Geometry: see drawing. Coordinates: mm, zero at the bounding-box minimum. A direction names the side the tool comes from. Round coordinates to 2 decimals unless told otherwise and drop trailing zeros. Loops run counter-clockwise (first coordinate to the right, second up) from the corner with the lowest first, then second, coordinate; pieces in that order, holes last.
(1) Cut plane A-A, the plane x = 4.75. Output: boundary loops of the cut face in (y, z).
(2) Draft query along X for the marked faces 3, 4, 5 and 6. Return one class per face: released by +X, released by -X, zero draft, split by the parting line, or undercut.
(3) First-contact query: pin 1 Ø1.5 at (x, y) = (9, 34.5) entering from -Z; pin 2 Ø5 at (x, y) = (8, 24.5) entering from +Z; pin 3 Ø1.5 at (x, z) = (8, 1.5) entering from +Y. Flat tips, straight axial feed; report the tip coordinate or a pass-through.
(4) Cut plane B-B, the plane z = 3.75. Output: boundary loops of the cut face in (x, y), and give its area (3 significant figures).
(5) Access query for the marked faces 1 and 2. Directions: +Z, -Z, +X, -X, +Y, -Y. A direction counts if a zero-diameter tool reaches every point of the face in a straight line with its end or side. Return the directions, or none.
(6) Line query: line 1 (Z direction, x = 3.25, y = 8); line 2 (X direction, y = 16.5, z = 4); line 3 (Z direction, x = 14.25, y = 33.5). Output: solid intervals per line, ascending.
(7) Cut plane D-D, the plane x = 14.75. Output: boundary loops of the cut face in (y, z).
(8) Cut plane C-C, the plane y = 35. Output: boundary loops of the cut face in (x, z), and give its area (3 significant figures).
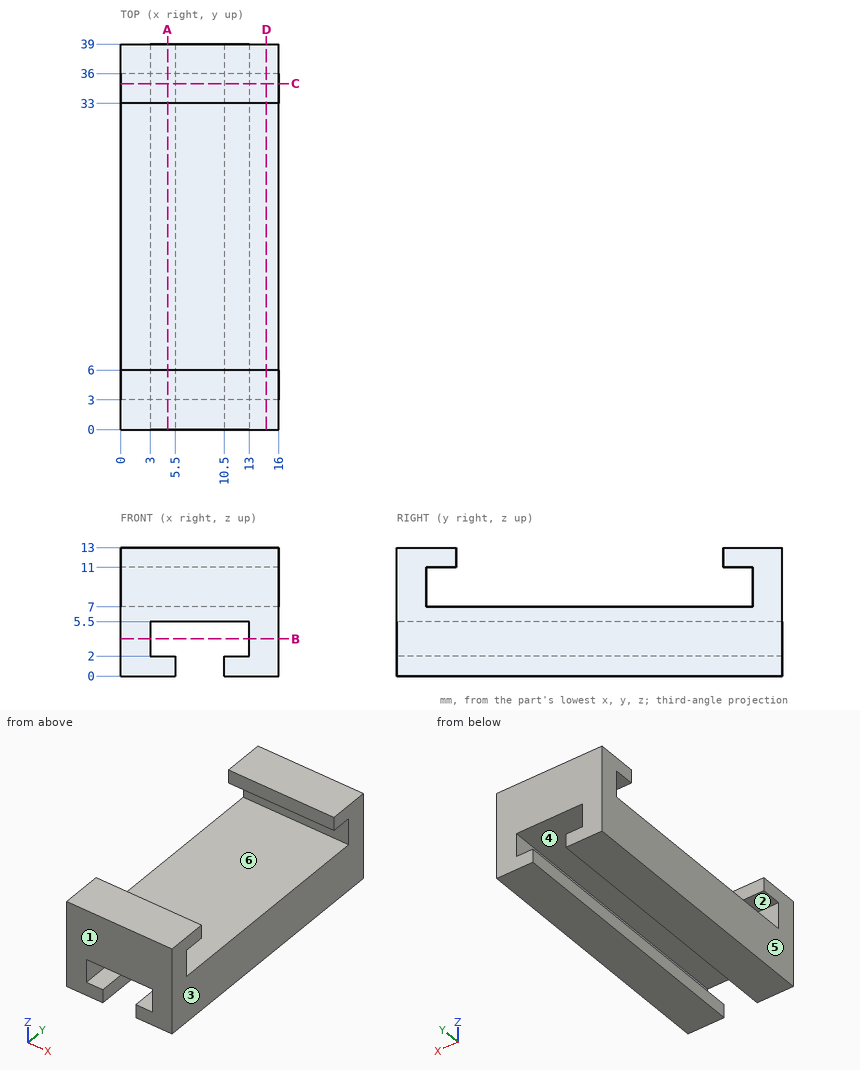
Reported:
1. outline: (0, 0) - (39, 0) - (39, 2) - (0, 2) - close; (0, 5.5) - (39, 5.5) - (39, 13) - (33, 13) - (33, 11) - (36, 11) - (36, 7) - (3, 7) - (3, 11) - (6, 11) - (6, 13) - (0, 13) - close
2. face 3: released by +X
2. face 4: undercut
2. face 5: released by -X
2. face 6: zero draft
3. pin 1: stops at z = 5.5
3. pin 2: stops at z = 7
3. pin 3: passes through
4. outline: (0, 0) - (3, 0) - (3, 39) - (0, 39) - close; (13, 0) - (16, 0) - (16, 39) - (13, 39) - close
4. area: 234 mm2
5. face 1: +Z, -Z, +X, -X, -Y
5. face 2: +X, -X
6. line 1: z = 0 to 2, 5.5 to 7
6. line 2: x = 0 to 3, 13 to 16
6. line 3: z = 0 to 7, 11 to 13
7. outline: (0, 0) - (39, 0) - (39, 13) - (33, 13) - (33, 11) - (36, 11) - (36, 7) - (3, 7) - (3, 11) - (6, 11) - (6, 13) - (0, 13) - close
8. outline: (0, 0) - (5.5, 0) - (5.5, 2) - (3, 2) - (3, 5.5) - (13, 5.5) - (13, 2) - (10.5, 2) - (10.5, 0) - (16, 0) - (16, 7) - (0, 7) - close; (0, 11) - (16, 11) - (16, 13) - (0, 13) - close
8. area: 99.0 mm2
